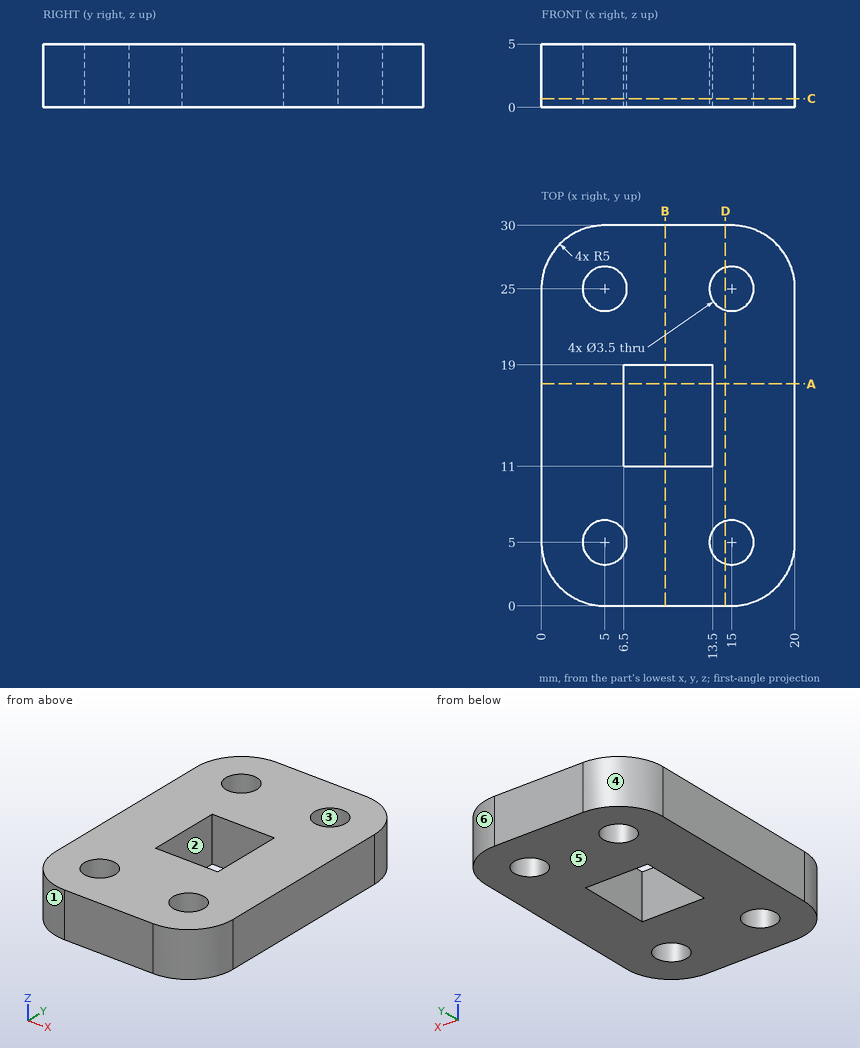
Geometry check sheet. Reference: drawing and pictorial views, mm from the part's lowest x, y, z. A direction names the side the tool comes from. Round coordinates to 2 decimals unless told otherwise and drop trailing zeros. Loops run counter-clockwise (first coordinate to the right, second up) from the corner with the lowest first, then second, coordinate; pieces in that order, holes last.
1. Set-up check for the marked faces 1 and 2: record each of +Z, -Z, +X, -X, +Y, -Y from which the full face is reachable in a straight line by a thin tool's end or side.
2. Sectioned sample at D-D on x = 14.5. Record the boundary of the cut face in (y, z).
3. Scan lines: probe 1 along Y at (x, z) = (7.75, 1.35); probe 2 along X at (y, z) = (4, 1.85); probe 3 along X at (y, z) = (5.5, 1.6). Record each from-to range of solid material in increasing order.
4. Mould release check, pull along X, two halves, no side actions. Record for the marked faces 3, 4, 5 and 6: released by +X, released by -X, zero draft, split by the parting line, or undercut.
5. Sectioned sample at C-C on z = 0.7. Record the boundary of the cut face in (x, y), and give its area (3 significant figures).
6. Sectioned sample at B-B on x = 9.75. Record the boundary of the cut face in (y, z).
7. Gauge pin test, flat end, axial feed: pin 1 Ø3 at (x, y) = (5, 25) entering from -Z. Record the tip position at first contact, or that the pin passes through.
8. Sectioned sample at A-A on y = 17.5. Record the boundary of the cut face in (x, z), and give its area (3 significant figures).
Recorded:
1. face 1: +Z, -Z, -X, -Y
1. face 2: +Z, -Z
2. outline: (0, 0) - (3.32, 0) - (3.32, 5) - (0, 5) - close; (6.68, 0) - (23.32, 0) - (23.32, 5) - (6.68, 5) - close; (26.68, 0) - (30, 0) - (30, 5) - (26.68, 5) - close
3. probe 1: y = 0 to 11, 19 to 30
3. probe 2: x = 0.1 to 3.56, 6.44 to 13.56, 16.44 to 19.9
3. probe 3: x = 0 to 3.32, 6.68 to 13.32, 16.68 to 20
4. face 3: undercut
4. face 4: released by -X
4. face 5: zero draft
4. face 6: released by +X
5. outline: (0, 5) arc R5 ccw to (5, 0) - (15, 0) arc R5 ccw to (20, 5) - (20, 25) arc R5 ccw to (15, 30) - (5, 30) arc R5 ccw to (0, 25) - close; hole circle Ø3.5 at (5, 5); hole circle Ø3.5 at (5, 25); hole (6.5, 11) - (13.5, 11) - (13.5, 19) - (6.5, 19) - close; hole circle Ø3.5 at (15, 5); hole circle Ø3.5 at (15, 25)
5. area: 484 mm2
6. outline: (0, 0) - (11, 0) - (11, 5) - (0, 5) - close; (19, 0) - (30, 0) - (30, 5) - (19, 5) - close
7. pin 1: passes through
8. outline: (0, 0) - (6.5, 0) - (6.5, 5) - (0, 5) - close; (13.5, 0) - (20, 0) - (20, 5) - (13.5, 5) - close
8. area: 65.0 mm2
